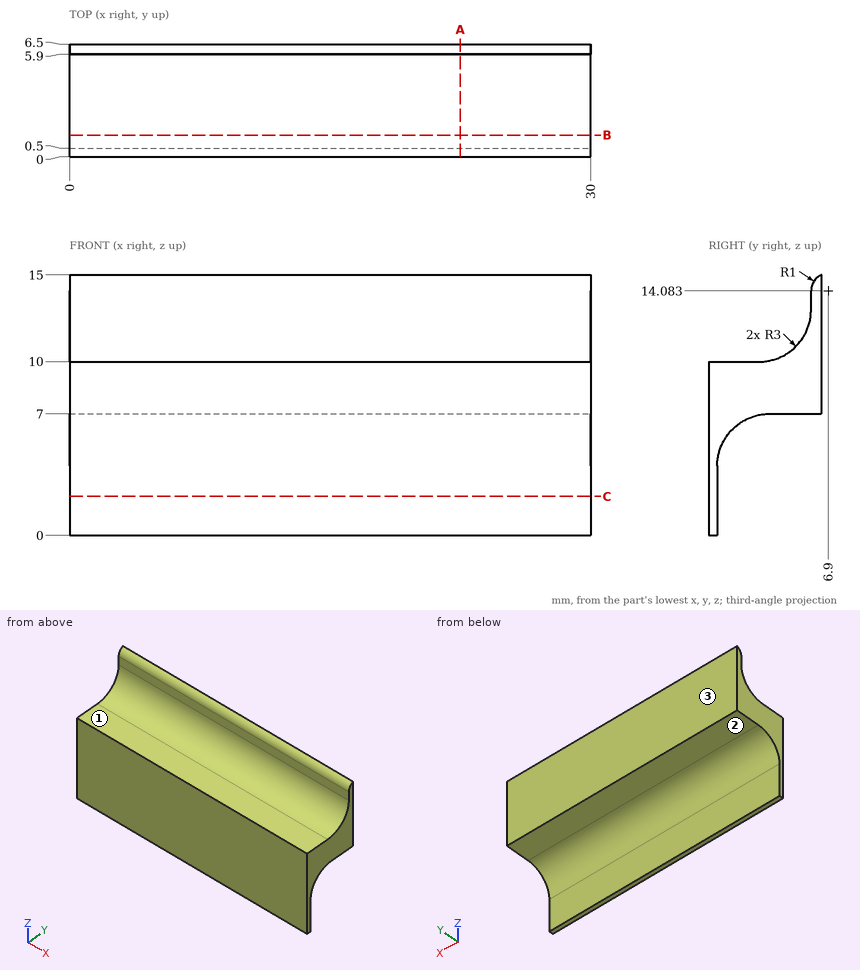
Geometry: see drawing. Coordinates: mm, zero at the bounding-box minimum. A direction names the side the tool comes from. Give positions to 0.01 mm unless a question says otherwise; leave off trailing zeros. Order: outer loops, then holes, each group sorted by start corner. A loop starts at its lowest first (then second) coordinate and runs counter-clockwise, first axis right, second up.
1. Line query: probe 1 along Y at (x, z) = (27.75, 13); probe 2 along Y at (x, z) = (9.5, 2.25); probe 3 along Z at (x, y) = (14, 3.25). Output: solid intervals per line, ascending.
Computed:
probe 1: y = 5.9 to 6.5
probe 2: y = 0 to 0.5
probe 3: z = 6.99 to 10.02
2. Cut plane C-C (z = 2.25). Return loops of the section in (x, y).
Computed:
outline: (0, 0) - (30, 0) - (30, 0.5) - (0, 0.5) - close
3. Set-up query: the marked faces 1, 2 and 3. Return all of +Z, -Z, +X, -X, +Y, -Y with unobstructed straight access to the full face (end or side cutting, diameter ignored); none if empty.
Computed:
face 1: +Z, +X, -X, -Y
face 2: -Z, +X, -X, +Y
face 3: +Z, -Z, +X, -X, +Y
4. Cut plane A-A (x = 22.5). Return loops of the section in (y, z).
Computed:
outline: (0, 0) - (0.5, 0) - (0.5, 4) arc R3 cw to (3.5, 7) - (6.5, 7) - (6.5, 15) arc R1 ccw to (5.9, 14.08) - (5.9, 13) arc R3 cw to (2.9, 10) - (0, 10) - close
5. Cut plane B-B (y = 1.25). Return loops of the section in (x, z) (1 decimal).
Computed:
outline: (0, 6) - (30, 6) - (30, 10) - (0, 10) - close
6. Pin query (flat end, axial travel): pin 1 Ø2 at (x, y) = (22.5, 5.5) entering from -Z; pin 2 Ø1.2 at (x, z) = (13.5, 2) entering from +Y; pin 3 Ø1.5 at (x, y) = (13.5, 2) entering from +Z; pin 4 Ø2 at (y, z) = (3.5, 13) entering from +X. Return the tip coordinate at first contact, or that it passes through.
Computed:
pin 1: stops at z = 7
pin 2: stops at y = 0.5
pin 3: stops at z = 10
pin 4: passes through
